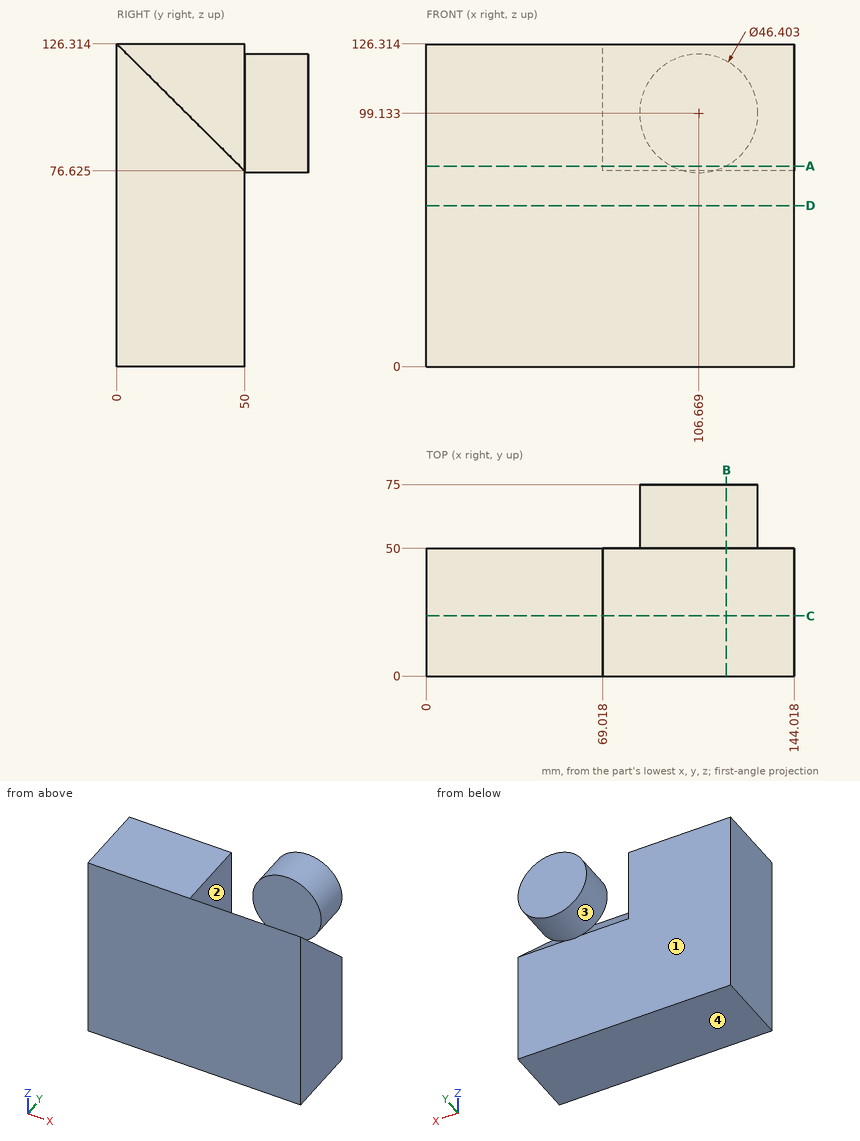
Geometry: see drawing. Coordinates: mm, zero at the bounding-box minimum. A direction names the side the tool comes from. Give positions to 0.01 mm unless a question says otherwise; leave off trailing zeros. Loops run counter-clockwise (first coordinate to the right, second up) from the corner with the lowest first, then second, coordinate; pieces in that order, holes last. Notation, with made-up numbers: (68.25, 34) -> (92.25, 34) arc R15 cw to (92.25, 57) -> close; hole circle Ø1 at (44.5, 29). An arc over 180 degrees is marked (long way). Use one line per item in the form item = value.
Item 1: Access query for the marked faces 1, 2, 3 and 4. Directions: +Z, -Z, +X, -X, +Y, -Y. A direction counts if a zero-diameter tool reaches every point of the face in a straight line with its end or side. Return the directions, or none.
A:
face_1 = -Z, -X, +Y
face_2 = +Z, +X, +Y
face_3 = +Y
face_4 = -Z, +X, -X, +Y, -Y
Item 2: Section query B-B on x = 117.5. Output: boundary loops of the cut face in (y, z) (1 decimal).
A:
outline = (0, 0) -> (50, 0) -> (50, 76.6) -> (0, 126.3) -> close; (50, 78.6) -> (75, 78.6) -> (75, 119.7) -> (50, 119.7) -> close
Item 3: Line query: probe 1 along X at (y, z) = (40.5, 116.5); probe 2 along Y at (x, z) = (20, 63.5); probe 3 along X at (y, z) = (61, 99.5). Output: solid intervals per line, ascending.
A:
probe_1 = 0 to 69.02
probe_2 = 0 to 50
probe_3 = 83.47 to 129.87
Item 4: Section query A-A on z = 78.5. Output: boundary loops of the cut face in (x, y).
A:
outline = (0, 0) -> (144.02, 0) -> (144.02, 48.11) -> (69.02, 48.11) -> (69.02, 50) -> (0, 50) -> close; (96.06, 50) -> (117.28, 50) -> (117.28, 75) -> (96.06, 75) -> close
Item 5: Section query C-C on y = 23.5. Output: boundary loops of the cut face in (x, z).
A:
outline = (0, 0) -> (144.02, 0) -> (144.02, 102.96) -> (69.02, 102.96) -> (69.02, 126.31) -> (0, 126.31) -> close
Item 6: Section query D-D on z = 63. Output: boundary loops of the cut face in (x, y).
A:
outline = (0, 0) -> (144.02, 0) -> (144.02, 50) -> (0, 50) -> close
Item 7: Pin query (flat end, axial travel): P1, Ø8, axis at x = 112, z = 23, coming from the -Y side; P2, Ø3, axis at x = 104.5, z = 42.5, coming from the +Y side; P3, Ø6, axis at y = 49, z = 108, coming from the +X side. Return the tip coordinate at first contact, or that it passes through.
A:
P1 = 0
P2 = 50
P3 = 129.07
